from build123d import *

# Parameters (mm, degrees)
SKETCH1_R           = 1.75
SKETCH1_R_2         = 1.8
BOSS_EXTRUDE1_DEPTH = 3


with BuildPart() as part:
    # Sketch1 → Boss-Extrude1 (new body)
    with BuildSketch(Plane.XY):
        with BuildLine():
            Line((126, 219), (126, 224))
            Line((126, 224), (147, 224))
            ThreePointArc((147, 224), (148.414213562, 224.585786438), (149, 226))
            Line((149, 226), (149, 332))
            ThreePointArc((149, 332), (148.414213562, 333.414213562), (147, 334))
            Line((147, 334), (-147, 334))
            ThreePointArc((-147, 334), (-148.414213562, 333.414213562), (-149, 332))
            Line((-149, 332), (-149, 226))
            ThreePointArc((-149, 226), (-148.414213562, 224.585786438), (-147, 224))
            Line((-147, 224), (-126, 224))
            Line((-126, 224), (-126, 219))
            Line((-126, 219), (-70, 219))
            Line((-70, 219), (70, 219))
            Line((70, 219), (126, 219))
        make_face()
        with Locations((136, 239)):
            Circle(SKETCH1_R, mode=Mode.SUBTRACT)
        with Locations((136, 319)):
            Circle(SKETCH1_R, mode=Mode.SUBTRACT)
        with Locations(Location((-136, 239, 0), (0, 0, 180))):
            Circle(SKETCH1_R, mode=Mode.SUBTRACT)
        with Locations(Location((-136, 319, 0), (0, 0, 180))):
            Circle(SKETCH1_R, mode=Mode.SUBTRACT)
        with Locations((-78.3, 324.25)):
            Circle(SKETCH1_R, mode=Mode.SUBTRACT)
        with Locations((-2.5, 321.5)):
            Circle(SKETCH1_R, mode=Mode.SUBTRACT)
        with Locations((-78.3, 284.25)):
            Circle(SKETCH1_R, mode=Mode.SUBTRACT)
        with Locations((-118.3, 324.25)):
            Circle(SKETCH1_R, mode=Mode.SUBTRACT)
        with Locations((-118.3, 284.25)):
            Circle(SKETCH1_R, mode=Mode.SUBTRACT)
        with Locations((-53.6, 324.25)):
            Circle(SKETCH1_R, mode=Mode.SUBTRACT)
        with Locations((-53.6, 284.25)):
            Circle(SKETCH1_R, mode=Mode.SUBTRACT)
        with Locations((-13.6, 324.25)):
            Circle(SKETCH1_R, mode=Mode.SUBTRACT)
        with Locations((-13.6, 284.25)):
            Circle(SKETCH1_R, mode=Mode.SUBTRACT)
        with Locations((71.3, 295.2)):
            Circle(SKETCH1_R, mode=Mode.SUBTRACT)
        with Locations((19.4, 288.5)):
            Circle(SKETCH1_R, mode=Mode.SUBTRACT)
        with Locations((19.4, 252.2)):
            Circle(SKETCH1_R, mode=Mode.SUBTRACT)
        with Locations((71.3, 252.2)):
            Circle(SKETCH1_R, mode=Mode.SUBTRACT)
        with Locations((39.5, 329.5)):
            Circle(SKETCH1_R, mode=Mode.SUBTRACT)
        with Locations((39.5, 299.5)):
            Circle(SKETCH1_R, mode=Mode.SUBTRACT)
        with Locations((92.5, 329.5)):
            Circle(SKETCH1_R, mode=Mode.SUBTRACT)
        with Locations((92.5, 299.5)):
            Circle(SKETCH1_R, mode=Mode.SUBTRACT)
        with Locations((8.54, 321.5)):
            Circle(SKETCH1_R, mode=Mode.SUBTRACT)
        with Locations((-2.5, 301.5)):
            Circle(SKETCH1_R, mode=Mode.SUBTRACT)
        with Locations((8.54, 301.5)):
            Circle(SKETCH1_R, mode=Mode.SUBTRACT)
        with Locations((-2.5, 271.5)):
            Circle(SKETCH1_R, mode=Mode.SUBTRACT)
        with Locations((8.54, 271.5)):
            Circle(SKETCH1_R, mode=Mode.SUBTRACT)
        with Locations((8.54, 251.5)):
            Circle(SKETCH1_R, mode=Mode.SUBTRACT)
        with Locations((-2.5, 251.5)):
            Circle(SKETCH1_R, mode=Mode.SUBTRACT)
        with Locations((105.977507251, 295.945086532)):
            Circle(SKETCH1_R_2, mode=Mode.SUBTRACT)
        with Locations((120.977507251, 295.945086532)):
            Circle(SKETCH1_R_2, mode=Mode.SUBTRACT)
    extrude(amount=BOSS_EXTRUDE1_DEPTH)


solid = part.part
The model under review builds one solid part; all positions refer to its coordinate system, in mm. Round coordinates to 2 decimals unless told otherwise and drop trailing zeros. Answer as a JSON object with one key per item and string values.
Item 1: Clearance check with a flat-ended pin moving along its axis: P1, Ø1.5, axis at y = 220.5, z = 1.5, coming from the -X side. State where the tip first meets the part, or that it passes through.
Check sheet entries:
{"P1": "x = -126"}
Item 2: For line 1 along X through (y, z) = (324.25, 1.4); line 2 along Y through (x, z) = (-136, 1.65); line 3 along Y through (x, z) = (8.54, 0.95), list the stretches that pass through material, from the lowest coordinate up.
Check sheet entries:
{"line 1": "-149 to -120.05, -116.55 to -80.05, -76.55 to -55.35, -51.85 to -15.35, -11.85 to 149", "line 2": "224 to 237.25, 240.75 to 317.25, 320.75 to 334", "line 3": "219 to 249.75, 253.25 to 269.75, 273.25 to 299.75, 303.25 to 319.75, 323.25 to 334"}
Item 3: We need section A-A, the plane z = 2.55. State how many separate pieces and enclosed holes the cut face has, and give its area (3 significant figures).
Check sheet entries:
{"separate pieces": "1", "enclosed holes": "30", "area": "33,700 mm2"}
